from build123d import *

# Parameters (mm, degrees)
F1_DEPTH = 40.2336
F0_R     = 10.16
F2_DEPTH = 15.875
F3_R     = 3.302


with BuildPart() as f1:
    # F0 (on Top) → F1 (new body)
    with BuildSketch(Plane.XY):
        with BuildLine():
            ThreePointArc((9.780705, -26.848993), (23.409552, -16.386686), (28.575, 0))
            ThreePointArc((28.575, 0), (23.409552, 16.386686), (9.780705, 26.848993))
            ThreePointArc((9.780705, 26.848993), (-28.575, 0), (9.780705, -26.848993))
        make_face()
        with BuildLine():
            ThreePointArc((-13.447765, -4.826), (-14.2875, 0), (-13.447765, 4.826))
            ThreePointArc((-13.447765, 4.826), (0, 14.2875), (13.447765, 4.826))
            Line((13.447765, 4.826), (18.5293, 4.826))
            Line((18.5293, 4.826), (18.5293, -4.826))
            Line((18.5293, -4.826), (13.447765, -4.826))
            ThreePointArc((13.447765, -4.826), (0, -14.2875), (-13.447765, -4.826))
        make_face(mode=Mode.SUBTRACT)
    extrude(amount=F1_DEPTH)

    # F0 (on Top) → F2 (join)
    with BuildSketch(Plane.XY):
        with BuildLine():
            ThreePointArc((9.780705, -26.848993), (23.409552, -16.386686), (28.575, 0))
            ThreePointArc((28.575, 0), (23.409552, 16.386686), (9.780705, 26.848993))
            ThreePointArc((9.780705, 26.848993), (-28.575, 0), (9.780705, -26.848993))
        make_face()
        with BuildLine():
            ThreePointArc((-13.447765, -4.826), (-14.2875, 0), (-13.447765, 4.826))
            ThreePointArc((-13.447765, 4.826), (0, 14.2875), (13.447765, 4.826))
            Line((13.447765, 4.826), (18.5293, 4.826))
            Line((18.5293, 4.826), (18.5293, -4.826))
            Line((18.5293, -4.826), (13.447765, -4.826))
            ThreePointArc((13.447765, -4.826), (0, -14.2875), (-13.447765, -4.826))
        make_face(mode=Mode.SUBTRACT)
        with BuildLine():
            ThreePointArc((9.780705, 26.848993), (23.409552, 16.386686), (28.575, 0))
            ThreePointArc((28.575, 0), (23.409552, -16.386686), (9.780705, -26.848993))
            Line((9.780705, -26.848993), (53.975, -19.05))
            ThreePointArc((53.975, -19.05), (73.025, 0), (53.975, 19.05))
            Line((53.975, 19.05), (9.780705, 26.848993))
        make_face()
        with Locations((53.975, 0)):
            Circle(F0_R, mode=Mode.SUBTRACT)
    extrude(amount=F2_DEPTH)

    # F3
    f3_edges = [f1.edges().sort_by_distance(p)[0] for p in [
        (-9.780705, 26.848993, 40.2336),
    ]]
    fillet(f3_edges, radius=F3_R)


solid = f1.part
Check sheet for the modelled part. Datum: model origin and axes. Units: mm. A direction names the side the tool comes from. Round coordinates to 2 decimals unless told otherwise and drop trailing zeros. Loops run counter-clockwise (first coordinate to the right, second up) from the corner with the lowest first, then second, coordinate; pieces in that order, holes last. Notation, with made-up numbers: M -7.75,34.25 L 47.25,34.25 A6 cw 47.25,39.25 Z; hole C 9,42.25 d6. An arc over 180 degrees is marked long. One line per item, written item: value.
(1) Sectioned sample at B-B, the plane z = 4. Count the separate pieces of the cut face and the enclosed holes in it, then the cut area to 3 significant figures.
Computed values:
separate pieces: 1
enclosed holes: 2
area: 3,420 mm^2
(2) Depth check by flat-ended pin: pin 1 Ø1.5 at (x, z) = (21, 23.5) entering from +Y; pin 2 Ø4 at (x, y) = (57, 11) entering from +Z (3 decimals); pin 3 Ø12 at (y, z) = (-7.5, 27.5) entering from -X. Enter the tip coordinate at first touch or a pass-through.
Computed values:
pin 1: stops at y = 20.16
pin 2: stops at z = 15.875
pin 3: stops at x = -28.54
(3) Release check for a two-part mould opening along Y. For faces 1 (the face through (31.6, -23, 7.8)), 2 (the face through (22, 0, 0)), 3 (the face through (16, 4.826, 20)) record: +Y half, -Y half, draft (parallel to the pull), parting line (faces both ways), or undercut.
Computed values:
face 1: -Y half
face 2: draft
face 3: undercut
(4) Sectioned sample at D-D, the plane x = 34. Record the cut outline in (y, z) (3 decimals).
Computed values:
outline: M -22.575,0 L 22.575,0 L 22.575,15.875 L -22.575,15.875 Z
(5) Access from +Z, -Z, +X, -X, +Y, -Y to the whole of each face (thin tool, end or side, straight path). Record for faces 4 (the face through (16, -4.826, 20)), 5 (the face through (73.02, -0.42, 7.83)).
Computed values:
face 4: +Z, -Z
face 5: +Z, -Z, +X
(6) Thickness scan on line 1 (Z direction, x = 55.5, y = 15.5) (3 decimals); line 2 (Y direction, x = -0.5, z = 12); line 3 (X direction, y = -8.5, z = 37). Record the ranges inside material, lowest first.
Computed values:
line 1: z = 0 to 15.875
line 2: y = -28.57 to -14.28, 14.28 to 28.57
line 3: x = -27.28 to -11.48, 11.48 to 27.28
